```python
from build123d import *

# Parameters (mm, degrees)
CROQUIS2_R              = 4.7625
SALIENTE_EXTRUIR1_DEPTH = 26.9875
CHAFL_N1_SIZE           = 0.396875
TAP_START               = 26.9875
CROQUIS3_R              = 2.0193
TAP_HOLE_1_DEPTH        = 19.05
TAP_START_2             = -7.9375
CROQUIS3_2_R            = 2.0193
TAP_HOLE_2_DEPTH        = 19.05


with BuildPart() as part:
    # Croquis2 → Saliente-Extruir1 (new, symmetric)
    with BuildSketch(Plane(origin=(0, 0, 0), x_dir=(1, 0, 0), z_dir=(0, 1, 0))):
        with Locations(Location((0, 0, 0), (0, 0, 270))):
            Circle(CROQUIS2_R)
    extrude(amount=SALIENTE_EXTRUIR1_DEPTH, both=True)

    # Chaflán1
    chafl_n1_edges = [part.edges().sort_by_distance(p)[0] for p in [
        (0, -26.9875, -4.7625),
        (0, 26.9875, -4.7625),
    ]]
    chamfer(chafl_n1_edges, length=CHAFL_N1_SIZE)

    # Croquis3 → Tap Hole 1 (cut)
    with BuildSketch(Plane(origin=(0, 0, 0), x_dir=(1, 0, 0), z_dir=(0, 1, 0)).offset(TAP_START)):
        with Locations(Location((0, 0, 0), (0, 0, 270))):
            Circle(CROQUIS3_R)
    extrude(amount=-TAP_HOLE_1_DEPTH, mode=Mode.SUBTRACT)

    # Croquis3<2> → Tap Hole 2 (cut)
    with BuildSketch(Plane(origin=(0, 0, 0), x_dir=(1, 0, 0), z_dir=(0, 1, 0)).offset(TAP_START_2)):
        with Locations(Location((0, 0, 0), (0, 0, 270))):
            Circle(CROQUIS3_2_R)
    extrude(amount=-TAP_HOLE_2_DEPTH, mode=Mode.SUBTRACT)


solid = part.part
```
Input: part model. Units: mm. Frame: model coordinates. A direction names the side the tool comes from. Round coordinates to 2 decimals unless told otherwise and drop trailing zeros. Write each loop counter-clockwise with the first axis right and the second up, starting at its lowest first coordinate (ties: lowest second). Pieces come first, ordered by that corner, then holes. Notation, with made-up numbers: M -38.75,17.5 L -20.75,17.5 A35 ccw -20.75,52.5 Z; hole C 54,-19.75 d4. An arc over 180 degrees is marked long. Write each question's results on one line, items separated by ' | '.
Q1. Section query A-A (z = 0). Return loops of the section in (x, y), and give its area (3 significant figures).
Results:
outline: M -4.76,-26.59 L -4.37,-26.99 L -2.02,-26.99 L -2.02,-7.94 L 2.02,-7.94 L 2.02,-26.99 L 4.37,-26.99 L 4.76,-26.59 L 4.76,26.59 L 4.37,26.99 L 2.02,26.99 L 2.02,7.94 L -2.02,7.94 L -2.02,26.99 L -4.37,26.99 L -4.76,26.59 Z | area: 360 mm^2
Q2. Access query for faces 1 (the face through (0, -7.938, 0)), 2 (the face through (-1, -26.988, 2)), 3 (the face through (0, 7.938, 0)). Directions: +Z, -Z, +X, -X, +Y, -Y. A direction counts if a zero-diameter tool reaches every point of the face in a straight line with its end or side. Return the directions, or none.
Results:
face 1: -Y | face 2: +Z, -Z, +X, -X, -Y | face 3: +Y
Q3. Section query B-B (x = 0). Return loops of the section in (y, z).
Results:
outline: M -26.99,-4.37 L -26.59,-4.76 L 26.59,-4.76 L 26.99,-4.37 L 26.99,-2.02 L 7.94,-2.02 L 7.94,2.02 L 26.99,2.02 L 26.99,4.37 L 26.59,4.76 L -26.59,4.76 L -26.99,4.37 L -26.99,2.02 L -7.94,2.02 L -7.94,-2.02 L -26.99,-2.02 Z
Q4. Draft query along Z for faces 4 (the face through (0.607, 17.596, 1.926)), 5 (the face through (-1, 26.988, 2)), 6 (the face through (-2.9, 0.37, -3.78)). Return one class per face: released by +Z, released by -Z, zero draft, split by the parting line, or undercut.
Results:
face 4: undercut | face 5: zero draft | face 6: split by the parting line
Q5. Section query C-C (y = 15). Return loops of the section in (x, z) (1 decimal).
Results:
outline: C 0,0 d9.5; hole C 0,0 d4
Q6. Pin query (flat end, axial travel): P1, Ø1.5, axis at y = 10.5, z = -1, coming from the -X side; P2, Ø4, axis at y = -17.5, z = 2.5, coming from the +X side; P3, Ø2, axis at x = 0.5, z = 0.5, coming from the +Y side; P4, Ø5, axis at x = 0, z = 0.5, coming from the -Y side. Return the tip coordinate at first contact, or that it passes through.
Results:
P1: stops at x = -4.76 | P2: stops at x = 4.74 | P3: stops at y = 7.94 | P4: stops at y = -26.99
Q7. Line query: line 1 along X through (y, z) = (-12.75, 0); line 2 along Z through (x, y) = (0.25, 17.5); line 3 along Z through (x, y) = (-1.75, 17). Output: solid intervals per line, ascending.
Results:
line 1: x = -4.76 to -2.02, 2.02 to 4.76 | line 2: z = -4.76 to -2, 2 to 4.76 | line 3: z = -4.43 to -1.01, 1.01 to 4.43
